from build123d import *

# Parameters (mm, degrees)
SKETCH_R        = 37
SKETCH_R_2      = 8
SKETCH_R_3      = 3
PAD_DEPTH       = 30
SKETCH006_R     = 12
SKETCH006_R_2   = 8
PAD001_DEPTH    = 4
SKETCH007_R     = 4.5
POCKET_DEPTH    = 7.2
PAD002_DEPTH    = 12
SKETCH009_R     = 6.75
PAD003_DEPTH    = 6.5
SKETCH010_R     = 4
PAD004_DEPTH    = 27
SKETCH011_R     = 26.25
SKETCH011_R_2   = 12
POCKET001_DEPTH = 1
SKETCH012_R     = 26
SKETCH012_R_2   = 12
POCKET002_DEPTH = 2
SKETCH013_R     = 12
POCKET003_DEPTH = 1


with BuildPart() as part:
    # Sketch → Pad (new body)
    with BuildSketch(Plane.XY):
        Circle(SKETCH_R)
        Circle(SKETCH_R_2, mode=Mode.SUBTRACT)
        with Locations((12.054528, 29.102205)):
            Circle(SKETCH_R_3, mode=Mode.SUBTRACT)
        with Locations((-29.102205, 12.054528)):
            Circle(SKETCH_R_3, mode=Mode.SUBTRACT)
        with Locations((-29.102205, -12.054528)):
            Circle(SKETCH_R_3, mode=Mode.SUBTRACT)
        with Locations((-12.054528, -29.102205)):
            Circle(SKETCH_R_3, mode=Mode.SUBTRACT)
        with Locations((29.102205, -12.054528)):
            Circle(SKETCH_R_3, mode=Mode.SUBTRACT)
        with Locations((29.102205, 12.054528)):
            Circle(SKETCH_R_3, mode=Mode.SUBTRACT)
        with Locations((-12.054528, 29.102205)):
            Circle(SKETCH_R_3, mode=Mode.SUBTRACT)
        with Locations((12.054528, -29.102205)):
            Circle(SKETCH_R_3, mode=Mode.SUBTRACT)
    extrude(amount=PAD_DEPTH)

    # Sketch006 → Pad001 (join)
    with BuildSketch(Plane.XY.offset(30)):
        Circle(SKETCH006_R)
        Circle(SKETCH006_R_2, mode=Mode.SUBTRACT)
    extrude(amount=PAD001_DEPTH)

    # Sketch007 (on Face3 of Pad001) → Pocket (cut)
    with BuildSketch(Plane.XY.offset(30)):
        with Locations((-29.102205, 12.054528)):
            Circle(SKETCH007_R)
        with Locations((29.102205, 12.054528)):
            Circle(SKETCH007_R)
        with Locations((12.054528, 29.102205)):
            Circle(SKETCH007_R)
        with Locations((-12.054528, 29.102205)):
            Circle(SKETCH007_R)
        with Locations((12.054528, -29.102205)):
            Circle(SKETCH007_R)
        with Locations((-29.102205, -12.054528)):
            Circle(SKETCH007_R)
        with Locations((-12.054528, -29.102205)):
            Circle(SKETCH007_R)
        with Locations((29.102205, -12.054528)):
            Circle(SKETCH007_R)
    extrude(amount=-POCKET_DEPTH, mode=Mode.SUBTRACT)

    # Sketch008 → Pad002 (join)
    with BuildSketch(Plane.XZ.offset(35)):
        Polygon((0, 23.082904), (-7, 19.041452), (-7, 10.958548), (0, 6.917096), (7, 10.958548), (7, 19.041452), align=None)
    extrude(amount=PAD002_DEPTH)

    # Sketch009 (on Face28 of Pad002) → Pad003 (join)
    with BuildSketch(Plane.XZ.offset(47)):
        with Locations((0, 15)):
            Circle(SKETCH009_R)
    extrude(amount=PAD003_DEPTH)

    # Sketch010 (on Face40 of Pad003) → Pad004 (join)
    with BuildSketch(Plane.XZ.offset(53.5)):
        with Locations((0, 15)):
            Circle(SKETCH010_R)
    extrude(amount=PAD004_DEPTH)

    # Sketch011 (on Face3 of Pad004) → Pocket001 (cut)
    with BuildSketch(Plane.XY.offset(30)):
        Circle(SKETCH011_R)
        Circle(SKETCH011_R_2, mode=Mode.SUBTRACT)
    extrude(amount=-POCKET001_DEPTH, mode=Mode.SUBTRACT)

    # Sketch012 → Pocket002 (cut)
    with BuildSketch(Plane.XY):
        Circle(SKETCH012_R)
        Circle(SKETCH012_R_2, mode=Mode.SUBTRACT)
    extrude(amount=POCKET002_DEPTH, mode=Mode.SUBTRACT)

    # Sketch013 → Pocket003 (cut)
    with BuildSketch(Plane.XY):
        Circle(SKETCH013_R)
    extrude(amount=POCKET003_DEPTH, mode=Mode.SUBTRACT)


solid = part.part
Geometry: final body of the model. Coordinates: model frame, mm. A direction names the side the tool comes from. Give positions to 0.01 mm unless a question says otherwise; leave off trailing zeros. Loops run counter-clockwise (first coordinate to the right, second up) from the corner with the lowest first, then second, coordinate; pieces in that order, holes last. Notation, with made-up numbers: (76.5, -16.75) -> (129.5, -16.75) arc R24 cw to (129.5, 1.25) -> close; hole circle Ø7 at (35, 65.25). An arc over 180 degrees is marked (long way). Put each result on its own line as item: value.
1. Cut plane B-B (z = 15). Count the separate pieces of the cut face and the enclosed holes in it, plus the area to 3 significant figures.
Taken from the geometry:
separate pieces: 1
enclosed holes: 9
area: 4,320 mm2
2. Ray query, line 1 along Y through (x, z) = (27, 5.5); line 2 along X through (y, z) = (-31, 28.5); line 3 along Y through (x, z) = (14, 20). Return the intervals inside material, ascending. Write a range as [from, to].
Taken from the geometry:
line 1: y = [-25.3, -14.19], [-9.91, 9.91], [14.19, 25.3]
line 2: x = [-20.2, -16.13], [-7.97, 7.97], [16.13, 20.2]
line 3: y = [-34.25, -31.39], [-26.82, 26.82], [31.39, 34.25]
3. Cut plane A-A (y = 0). Return the cut outline in (x, z), plus the area to 3 significant figures.
Taken from the geometry:
outline: (-37, 0) -> (-26, 0) -> (-26, 2) -> (-12, 2) -> (-12, 1) -> (-8, 1) -> (-8, 34) -> (-12, 34) -> (-12, 29) -> (-26.25, 29) -> (-26.25, 30) -> (-37, 30) -> close; (8, 1) -> (12, 1) -> (12, 2) -> (26, 2) -> (26, 0) -> (37, 0) -> (37, 30) -> (26.25, 30) -> (26.25, 29) -> (12, 29) -> (12, 34) -> (8, 34) -> close
area: 1,680 mm2
4. Pin query (flat end, axial travel): P1, Ø1, axis at y = 3.5, z = 9, coming from the +X side; P2, Ø5.5, axis at x = -12.05, y = -29.1, coming from the +Z side; P3, Ø1, axis at x = 5.5, z = 24, coming from the -Y side; P4, Ø7, axis at x = 12.05, y = 29.1, coming from the +Z side. Return the tip coordinate at first contact, or that it passes through.
Taken from the geometry:
P1: stops at x = 36.88
P2: passes through
P3: stops at y = -36.66
P4: stops at z = 22.8
5. Pull-direction query (X, two-part tool) for faces 1 (the flat face through (-25, 9, 30)), 2 (the cylindrical face through (11.469, 33.564, 26.45)), 3 (the flat face through (-7, -42, 15)), 4 (the cylindrical face through (11.47, -24.64, 26.45)); classes: released by +X, released by -X, zero draft, split by the parting line, or undercut.
Taken from the geometry:
face 1: zero draft
face 2: undercut
face 3: released by -X
face 4: undercut
6. Set-up query: faces 5 (the cylindrical face through (24.607, -11.857, 26.45)), 6 (the flat face through (3.45, -41.59, 8.91)), 7 (the cylindrical face through (-0.521, -66.811, 18.966)). Return all of +Z, -Z, +X, -X, +Y, -Y with unobstructed straight access to the full face (end or side cutting, diameter ignored); none if empty.
Taken from the geometry:
face 5: +Z
face 6: -Z, +X, -Y
face 7: -Y
7. Cut plane C-C (x = -19). Return the cut outline in (y, z).
Taken from the geometry:
outline: (-31.75, 0) -> (-17.75, 0) -> (-17.75, 2) -> (17.75, 2) -> (17.75, 0) -> (31.75, 0) -> (31.75, 30) -> (18.11, 30) -> (18.11, 29) -> (-18.11, 29) -> (-18.11, 30) -> (-31.75, 30) -> close
